For this review, take the finished solid that the model builds, in its own axes (mm). A direction names the side the tool comes from. Round coordinates to 2 decimals unless told otherwise and drop trailing zeros. Write each loop counter-clockwise with the first axis right and the second up, starting at its lowest first coordinate (ties: lowest second). Pieces come first, ordered by that corner, then holes. Notation, with made-up numbers: M -35,-17.75 L 3,-17.75 A28 cw 3,3.25 Z; hole C 22,46 d1. An arc over 180 degrees is marked long. Use one line per item in the form item = value. Start each with the question number.
Item 1: For line 1 (Z direction, x = 15, y = 1.5); line 2 (Y direction, x = 7.5, z = -42.5); line 3 (Z direction, x = 53, y = 0.5), list the stretches that pass through material, from the lowest coordinate up. Write a range as [from, to].
Item 2: For faces 5 (the cylindrical face through (11.484, 16.265, 26.989)), 6 (the flat face through (13, -13, -88.771)), 7 (the cylindrical face through (32.172, -1.455, -4.273)), 8 (the flat face through (9, 15.57, -32)), 9 (the flat face through (-4, 10.87, -22)), list the 3-axis set-ups (+Z, -Z, +X, -X, +Y, -Y) from which the entire face can be reached by the end or side of a thin tool; tool diameter is ignored.
Item 3: Add section D-D (x = 12.7). Count the separate pieces of the cut face and the enclosed holes in it, and give its area (3 significant figures).
Item 4: Draft analysis for pull direction X (two halves, no side actions). For faces 1 (the flat face through (-0.238, 4, -20)), 2 (the flat face through (0, -12, -53)), 3 (the flat face through (13, -14.331, 62)), 4 (the flat face through (-4.1, 1.8, -14.596)), state which applies: released by +X, released by -X, zero draft, split by the parting line, or undercut.
Item 5: Add section B-B (z = 25). State the section outline as (x, y) points.
Item 6: For P1, Ø14, axis at x = 10, z = -32, coming from the -Y side; P2, Ø5, axis at x = 12.7, z = -31.79, coming from the -Y side; P3, Ø14.5, axis at x = 12.7, z = -79.42, coming from the +Y side; P4, Ø3, axis at x = 26.5, z = -1, coming from the -Y side, all flat-tipped, find the tip position at first contact; note any pin that passes through.
Item 7: Add section C-C (y = 8). State the section outline as (x, z) points (1 decimal), and give its area (3 significant figures).
Item 8: Add section A-A (x = 32.5). State the section outline as (y, z) points (3 decimals), and give its area (3 significant figures).
from build123d import *

# Parameters (mm, degrees)
BOSS_EXTRUDE2_DEPTH = 25.4
SKETCH5_R           = 6.35
CUT_EXTRUDE3_DEPTH  = 25.4
SKETCH6_R           = 6.35
CUT_EXTRUDE4_DEPTH  = 25.4
SKETCH7_R           = 3.175
CUT_EXTRUDE5_DEPTH  = 3.175
SKETCH8_R           = 3.175
CUT_EXTRUDE6_DEPTH  = 3.175
BOSS_EXTRUDE3_DEPTH = 5
BOSS_EXTRUDE4_DEPTH = 3.175
SKETCH12_W          = 6.35
SKETCH12_H          = 12.7
CUT_EXTRUDE7_DEPTH  = 74.175
BOSS_EXTRUDE5_DEPTH = 45


with BuildPart() as part:
    # Sketch4 → Boss-Extrude2 (new body)
    with BuildSketch(Plane(origin=(0, 0, 0), x_dir=(0, 0, -1), z_dir=(1, 0, 0))):
        with BuildLine():
            Line((-95.034446017, -11.155981989), (-95.034446017, -14.330981989))
            Line((-95.034446017, -14.330981989), (-28.199126576, -14.330981989))
            Line((-28.199126576, -14.330981989), (-11.780407797, 2.08773679))
            ThreePointArc((-11.780407797, 2.08773679), (3.868526207, -4.634940512), (19.517460211, 2.08773679))
            Line((19.517460211, 2.08773679), (35.93617899, -14.330981989))
            Line((35.93617899, -14.330981989), (88.77149843, -14.330981989))
            Line((88.77149843, -14.330981989), (88.77149843, -11.155981989))
            Line((88.77149843, -11.155981989), (37.251307051, -11.155981989))
            Line((37.251307051, -11.155981989), (21.536971904, 4.558353157))
            ThreePointArc((21.536971904, 4.558353157), (24.227085542, 9.797952879), (25.399969977, 15.569820752))
            Line((25.399969977, 15.569820752), (38.143526207, 15.569820752))
            Line((38.143526207, 15.569820752), (38.143526207, 16.940059488))
            Line((38.143526207, 16.940059488), (22.268526207, 16.940059488))
            ThreePointArc((22.268526207, 16.940059488), (3.868526207, -1.459940512), (-14.531473793, 16.940059488))
            Line((-14.531473793, 16.940059488), (-30.406473793, 16.940059488))
            Line((-30.406473793, 16.940059488), (-30.406473793, 15.569820752))
            Line((-30.406473793, 15.569820752), (-17.662917563, 15.569820752))
            ThreePointArc((-17.662917563, 15.569820752), (-16.490033128, 9.797952879), (-13.79991949, 4.558353157))
            Line((-13.79991949, 4.558353157), (-29.514254637, -11.155981989))
            Line((-29.514254637, -11.155981989), (-95.034446017, -11.155981989))
        make_face()
    extrude(amount=BOSS_EXTRUDE2_DEPTH)

    # Sketch5 → Cut-Extrude3 (cut)
    with BuildSketch(Plane(origin=(0, -11.155981989, 0), x_dir=(1, 0, 0), z_dir=(0, 1, 0))):
        with Locations(Location((12.7, -85.684446017, 0), (0, 0, 270))):
            Circle(SKETCH5_R)
    extrude(amount=-CUT_EXTRUDE3_DEPTH, mode=Mode.SUBTRACT)

    # Sketch6 → Cut-Extrude4 (cut)
    with BuildSketch(Plane(origin=(0, -11.155981989, 0), x_dir=(1, 0, 0), z_dir=(0, 1, 0))):
        with Locations(Location((12.7, 79.42149843, 0), (0, 0, 270))):
            Circle(SKETCH6_R)
    extrude(amount=-CUT_EXTRUDE4_DEPTH, mode=Mode.SUBTRACT)

    # Sketch7 → Cut-Extrude5 (cut)
    with BuildSketch(Plane(origin=(0, 16.940059488, 0), x_dir=(1, 0, 0), z_dir=(0, 1, 0))):
        with Locations(Location((12.7, -24.056473793, 0), (0, 0, 270))):
            Circle(SKETCH7_R)
    extrude(amount=-CUT_EXTRUDE5_DEPTH, mode=Mode.SUBTRACT)

    # Sketch8 → Cut-Extrude6 (cut)
    with BuildSketch(Plane(origin=(0, 16.940059488, 0), x_dir=(1, 0, 0), z_dir=(0, 1, 0))):
        with Locations(Location((12.7, 31.793526207, 0), (0, 0, 270))):
            Circle(SKETCH8_R)
    extrude(amount=-CUT_EXTRUDE6_DEPTH, mode=Mode.SUBTRACT)

    # Sketch10 → Boss-Extrude3 (add)
    with BuildSketch(Plane.ZY):
        with BuildLine():
            Line((-22.268526207, 16.940059488), (-29.184168721, 16.940059488))
            ThreePointArc((-29.184168721, 16.940059488), (-29.174889499, 16.254688903), (-29.147058635, 15.569820752))
            Line((-29.147058635, 15.569820752), (-25.399969977, 15.569820752))
            ThreePointArc((-25.399969977, 15.569820752), (-24.227085542, 9.797952879), (-21.536971904, 4.558353157))
            Line((-21.536971904, 4.558353157), (-24.216513217, 1.878811845))
            ThreePointArc((-24.216513217, 1.878811845), (-23.228268183, 0.628034888), (-22.163262525, -0.558065525))
            Line((-22.163262525, -0.558065525), (-19.517460211, 2.08773679))
            ThreePointArc((-19.517460211, 2.08773679), (-3.868526207, -4.634940512), (11.780407797, 2.08773679))
            Line((11.780407797, 2.08773679), (14.426210111, -0.558065525))
            ThreePointArc((14.426210111, -0.558065525), (15.491215769, 0.628034888), (16.479460803, 1.878811845))
            Line((16.479460803, 1.878811845), (13.79991949, 4.558353157))
            ThreePointArc((13.79991949, 4.558353157), (16.490033128, 9.797952879), (17.662917563, 15.569820752))
            Line((17.662917563, 15.569820752), (21.410006221, 15.569820752))
            ThreePointArc((21.410006221, 15.569820752), (21.437837085, 16.254688903), (21.447116307, 16.940059488))
            Line((21.447116307, 16.940059488), (14.531473793, 16.940059488))
            ThreePointArc((14.531473793, 16.940059488), (-3.868526207, -1.459940512), (-22.268526207, 16.940059488))
        make_face()
    extrude(amount=BOSS_EXTRUDE3_DEPTH)

    # Sketch11 → Boss-Extrude4 (add)
    with BuildSketch(Plane.ZY.offset(5)):
        with BuildLine():
            Line((21.297794872, 16.940059488), (-29.034847286, 16.940059488))
            ThreePointArc((-29.034847286, 16.940059488), (-29.025512905, 16.254685909), (-28.997516686, 15.569820752))
            Line((-28.997516686, 15.569820752), (-25.399969977, 15.569820752))
            ThreePointArc((-25.399969977, 15.569820752), (-24.227085542, 9.797952879), (-21.536971904, 4.558353157))
            Line((-21.536971904, 4.558353157), (-24.109749596, 1.985575465))
            ThreePointArc((-24.109749596, 1.985575465), (-23.122328229, 0.734047506), (-22.057650024, -0.452453023))
            Line((-22.057650024, -0.452453023), (-19.517460211, 2.08773679))
            ThreePointArc((-19.517460211, 2.08773679), (-3.868526207, -4.634940512), (11.780407797, 2.08773679))
            Line((11.780407797, 2.08773679), (14.32059761, -0.452453023))
            ThreePointArc((14.32059761, -0.452453023), (15.385275816, 0.734047506), (16.372697182, 1.985575465))
            Line((16.372697182, 1.985575465), (13.79991949, 4.558353157))
            ThreePointArc((13.79991949, 4.558353157), (16.490033128, 9.797952879), (17.662917563, 15.569820752))
            Line((17.662917563, 15.569820752), (21.260464272, 15.569820752))
            ThreePointArc((21.260464272, 15.569820752), (21.288460491, 16.254685909), (21.297794872, 16.940059488))
        make_face()
    extrude(amount=BOSS_EXTRUDE4_DEPTH)

    # Sketch12 → Cut-Extrude7 (cut)
    with BuildSketch(Plane(origin=(0, 0, -88.77149843), x_dir=(-1, 0, 0), z_dir=(0, 0, -1))):
        with Locations((3.4125, 4.519997663)):
            Rectangle(SKETCH12_W, SKETCH12_H)
    extrude(amount=-CUT_EXTRUDE7_DEPTH, mode=Mode.SUBTRACT)

    # Sketch13 → Boss-Extrude5 (add)
    with BuildSketch(Plane(origin=(25.4, 0, 0), x_dir=(0, 0, -1), z_dir=(1, 0, 0))):
        with BuildLine():
            Line((-14.531473793, 16.940059488), (-17.706473793, 16.940059488))
            ThreePointArc((-17.706473793, 16.940059488), (-17.695581986, 16.254594073), (-17.662917563, 15.569820752))
            ThreePointArc((-17.662917563, 15.569820752), (-16.490033128, 9.797952879), (-13.79991949, 4.558353157))
            ThreePointArc((-13.79991949, 4.558353157), (-12.835902363, 3.285657591), (-11.780407797, 2.08773679))
            ThreePointArc((-11.780407797, 2.08773679), (3.868526207, -4.634940512), (19.517460211, 2.08773679))
            ThreePointArc((19.517460211, 2.08773679), (20.572954777, 3.285657591), (21.536971904, 4.558353157))
            ThreePointArc((21.536971904, 4.558353157), (24.227085542, 9.797952879), (25.399969977, 15.569820752))
            ThreePointArc((25.399969977, 15.569820752), (25.4326344, 16.254594073), (25.443526207, 16.940059488))
            Line((25.443526207, 16.940059488), (22.268526207, 16.940059488))
            ThreePointArc((22.268526207, 16.940059488), (3.868526207, -1.459940512), (-14.531473793, 16.940059488))
        make_face()
    extrude(amount=BOSS_EXTRUDE5_DEPTH)


solid = part.part
Calculated:
q1.line_1 = [-24.6, -20.11], [-18.94, -13.88], [6.14, 11.2], [12.37, 16.86]
q1.line_2 = [-14.33, -11.16]
q1.line_3 = [-17.84, -12.13], [4.39, 10.1]
q2.face_5 = +Y
q2.face_6 = -Z, +X, -X, +Y, -Y
q2.face_7 = +X, +Y
q2.face_8 = -Z, +X, -X
q2.face_9 = -Z, -Y
q3.separate_pieces = 5
q3.enclosed_holes = 0
q3.area = 656 mm^2
q4.face_1 = undercut
q4.face_2 = released by -X
q4.face_3 = zero draft
q4.face_4 = undercut
q5.outline = M 0,-11.13 L 25.4,-11.13 L 25.4,-6.64 L 0,-6.64 Z; M 0,15.57 L 9.67,15.57 L 9.67,16.94 L 0,16.94 Z; M 15.73,15.57 L 25.4,15.57 L 25.4,16.94 L 15.73,16.94 Z
q6.P1 = -14.33
q6.P2 = -12.68
q6.P3 = -11.16
q6.P4 = -4.59
q7.outline = M -8.2,-23.5 L -6.6,-23.5 L -6.6,-14.6 L -5,-14.6 L -5,12.2 L 70.4,12.2 L 70.4,15.8 L -8.2,15.8 Z; M -0.2,-23.5 L 70.4,-23.5 L 70.4,-20 L -0.2,-20 Z
q7.area = 629 mm^2
q8.outline = M 16.94,-25.444 L 16.94,-22.269 A18.4 cw 16.94,14.531 L 16.94,17.706 A21.575 ccw Z
q8.area = 199 mm^2
